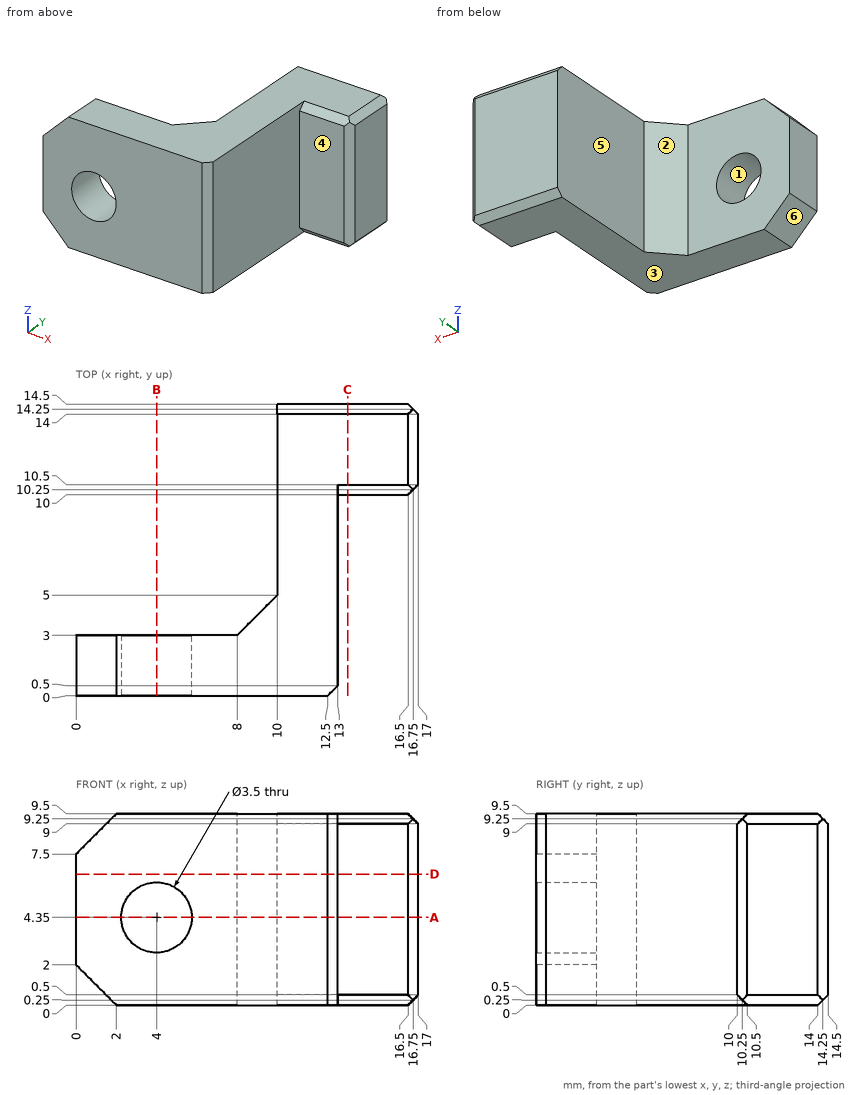
Geometry: see drawing. Coordinates: mm, zero at the bounding-box minimum. A direction names the side the tool comes from. Coordinates: 2 decimals unless noted, no trailing zeros. Loops run counter-clockwise (first coordinate to the right, second up) from the corner with the lowest first, then second, coordinate; pieces in that order, holes last. Notation, with made-up numbers: M -5,30.5 L 9,30.5 A25 cw 9,44.5 Z; hole C 60.5,11.25 d11. An arc over 180 degrees is marked long. Answer in a Markdown table with one row per item.
1. Section D-D, the plane z = 6.5. Output: boundary loops of the cut face in (x, y).
Response:
| item | result |
|---|---|
| outline | M 0,0 L 12.5,0 L 13,0.5 L 13,10 L 16.5,10 L 17,10.5 L 17,14 L 16.5,14.5 L 10,14.5 L 10,5 L 8,3 L 0,3 Z |
2. Reachability of the marked faces 4, 5 and 6 from +Z, -Z, +X, -X, +Y, -Y: full face, straight path, thin tool, end or side. Return the list, or none.
Response:
| item | result |
|---|---|
| face 4 | +Z, -Z, +X, -Y |
| face 5 | +Z, -Z, -X, +Y |
| face 6 | -Z, -X, +Y, -Y |
3. Draft query along X for the marked faces 1, 2 and 3. Return one class per face: pulls with the +X half, pulls with the -X half, needs draft (parallel to the pull), parting line crosses it, or undercut.
Response:
| item | result |
|---|---|
| face 1 | undercut |
| face 2 | pulls with the -X half |
| face 3 | needs draft |
4. Section A-A, the plane z = 4.35. Output: boundary loops of the cut face in (x, y).
Response:
| item | result |
|---|---|
| outline | M 0,0 L 2.25,0 L 2.25,3 L 0,3 Z; M 5.75,0 L 12.5,0 L 13,0.5 L 13,10 L 16.5,10 L 17,10.5 L 17,14 L 16.5,14.5 L 10,14.5 L 10,5 L 8,3 L 5.75,3 Z |
5. Section C-C, the plane x = 13.5. Output: boundary loops of the cut face in (y, z).
Response:
| item | result |
|---|---|
| outline | M 10,0.5 L 10.5,0 L 14,0 L 14.5,0.5 L 14.5,9 L 14,9.5 L 10.5,9.5 L 10,9 Z |
6. Section B-B, the plane x = 4. Output: boundary loops of the cut face in (y, z), then the cut area to 3 significant figures.
Response:
| item | result |
|---|---|
| outline | M 0,0 L 3,0 L 3,2.6 L 0,2.6 Z; M 0,6.1 L 3,6.1 L 3,9.5 L 0,9.5 Z |
| area | 18.0 mm2 |
7. First-contact query: pin 1 (4 mm diameter, centred on x = 13.5, z = 4, fed in from -Y); pin 2 (1.5 mm diameter, centred on x = 4, z = 6.5, fed in from +Y). Flat tips, straight axial feed; report the tip coordinate or a pass-through.
Response:
| item | result |
|---|---|
| pin 1 | stops at y = 0 |
| pin 2 | stops at y = 3 |
8. Material intervals for line 1 (Z direction, x = 4, y = 2.25); line 2 (X direction, y = 8.5, z = 0.5); line 3 (Y direction, x = 13.5, z = 3.25), sorted ascending.
Response:
| item | result |
|---|---|
| line 1 | z = 0 to 2.6, 6.1 to 9.5 |
| line 2 | x = 10 to 13 |
| line 3 | y = 10 to 14.5 |
